from build123d import *

# Parameters (mm, degrees)
F0_W      = 20
F0_H      = 20
F1_DEPTH  = 65
F0_R      = 15
F1_FACE_W = 20
F1_FACE_H = 20
F2_DEPTH  = 3
F3_R      = 10
F4_DEPTH  = 40.5
F6_D      = 5
F6_DEPTH  = 15
F6_TIP    = 1.5021515476
F7_SIZE   = 1
F9_D      = 6
F10_SIZE  = 2
F11_R     = 5


with BuildPart() as f1:
    # F0 (on Front) → F1 (new body)
    with BuildSketch(Plane.XZ):
        Rectangle(F0_W, F0_H)
    extrude(amount=F1_DEPTH)

    # F0 (on Front) + F1_face (on face) → F2 (join)
    with BuildSketch(Plane.XZ):
        Circle(F0_R)
        Rectangle(F0_W, F0_H, mode=Mode.SUBTRACT)
        Rectangle(F0_W, F0_H)
    with BuildSketch(Plane(origin=(0, 0, 0), x_dir=(1, 0, 0), z_dir=(0, 1, 0))):
        Rectangle(F1_FACE_W, F1_FACE_H)
    extrude(amount=-F2_DEPTH, dir=(0, -1, 0))

    # F3 (on face) → F4 (join)
    with BuildSketch(Plane(origin=(0, 3, 0), x_dir=(-1, 0, 0), z_dir=(0, 1, 0))):
        Circle(F3_R)
    extrude(amount=F4_DEPTH)

    # F6
    with Locations(Plane(origin=(0, 43.5, 0), x_dir=(-1, 0, 0), z_dir=(0, 1, 0))):
        with Locations((0, 0)):
            Hole(F6_D / 2, depth=F6_DEPTH)
            with Locations((0, 0, -(F6_DEPTH + F6_TIP / 2))):  # 118° drill point
                Cone(0, F6_D / 2, F6_TIP, mode=Mode.SUBTRACT)

    # F7
    f7_edges = [f1.edges().sort_by_distance(p)[0] for p in [
        (10, 43.5, 0),
    ]]
    chamfer(f7_edges, length=F7_SIZE)

    # F9 (through all)
    with Locations(Plane.XY.offset(10)):
        with Locations((0, -13), (0, -57)):
            Hole(F9_D / 2)

    # F10
    f10_edges = [f1.edges().sort_by_distance(p)[0] for p in [
        (0, -65, 10),
        (-10, -32.5, 10),
        (10, -32.5, 10),
    ]]
    chamfer(f10_edges, length=F10_SIZE)

    # F11
    f11_edges = [f1.edges().sort_by_distance(p)[0] for p in [
        (-10, -65, -1),
        (10, -65, -1),
    ]]
    fillet(f11_edges, radius=F11_R)


solid = f1.part
Part model, mm, in its own coordinate system. A direction names the side the tool comes from. Coordinates: 2 decimals unless noted, no trailing zeros. Loops run counter-clockwise (first coordinate to the right, second up) from the corner with the lowest first, then second, coordinate; pieces in that order, holes last. Notation, with made-up numbers: (11.5, -6.75) -> (17.5, -6.75) arc R12 ccw to (17.5, -0.75) -> close; hole circle Ø5 at (86.5, 44.25). An arc over 180 degrees is marked (long way). Use a Markdown table: item, result. Add a question column.
Item 1: Band-saw the part on B-B on y = 30.5. Write the cut outline in (x, z), plus the area to 3 significant figures.
Item 2: Which spindle directions (+Z, -Z, +X, -X, +Y, -Y) get a long thin tool onto all of the face, cutting with end or side? Do faces 1 (the flat face through (-11, 0, 1)), 2 (the flat face through (9, -31, 9)), 3 (the flat face through (-10, -30, -1)), 4 (the cylindrical face through (2.17, 22.47, -9.76)), 5 (the flat face through (0, -31, 10)). Say none if no direction does.
Item 3: Pull direction Y, two halves, no side cores. Call faces 6 (the cylindrical face through (0, -54, 0)), 7 (the flat face through (-9, -31, 9)), 8 (the cylindrical face through (-9, -63, 0)): +Y half, -Y half, draft (parallel to the pull), parting line (faces both ways), or undercut.
Item 4: Band-saw the part on A-A on y = -13. Write the cut outline in (x, z).
Item 5: Probe probe 1 along Y at (x, z) = (0, -5.5); probe 2 along Z at (x, y) = (0, 32.5); probe 3 along Y at (x, z) = (-2.75, -2.25). List the from-to ranges inside material, lowest first.
Item 6: Band-saw the part on C-C on z = -7.5. Give the number of separate pieces and of enclosed holes in the cut face, plus the area to 3 significant figures.
Item 7: Flat gauge pins, fed straight in: P1, Ø1.5, axis at y = -3.5, z = -1, coming from the +X side; P2, Ø12, axis at y = -1.5, z = -1.5, coming from the +X side; P3, Ø5, axis at x = 3, y = -32, coming from the +Z side; P4, Ø4, axis at x = 0, z = 0, coming from the +Y side. Where does each tip first touch, or does it go through?
Item 8: Band-saw the part on D-D on x = -11. Write the cut outline in (y, z).
Geometry says:
| question | item | result |
|---|---|---|
| 1 | outline | circle Ø20 at (0, 0); hole circle Ø5 at (0, 0) |
| 1 | area | 295 mm² |
| 2 | face 1 | -Y |
| 2 | face 2 | +Z, +X, -Y |
| 2 | face 3 | +Z, -Z, -X, -Y |
| 2 | face 4 | +Y |
| 2 | face 5 | +Z, +X, -X, -Y |
| 3 | face 6 | undercut |
| 3 | face 7 | draft |
| 3 | face 8 | -Y half |
| 4 | outline | (-10, -10) -> (-3, -10) -> (-3, 10) -> (-8, 10) -> (-10, 8) -> close; (3, -10) -> (10, -10) -> (10, 8) -> (8, 10) -> (3, 10) -> close |
| 5 | probe 1 | -65 to -60, -54 to -16, -10 to 43.5 |
| 5 | probe 2 | -10 to -2.5, 2.5 to 10 |
| 5 | probe 3 | -65 to -58.2, -55.8 to -14.2, -11.8 to 43.5 |
| 6 | separate pieces | 1 |
| 6 | enclosed holes | 2 |
| 6 | area | 1,840 mm² |
| 7 | P1 | x = 10 |
| 7 | P2 | x = 15 |
| 7 | P3 | z = 10 |
| 7 | P4 | y = 28.2 |
| 8 | outline | (0, -10.2) -> (3, -10.2) -> (3, 10.2) -> (0, 10.2) -> close |
